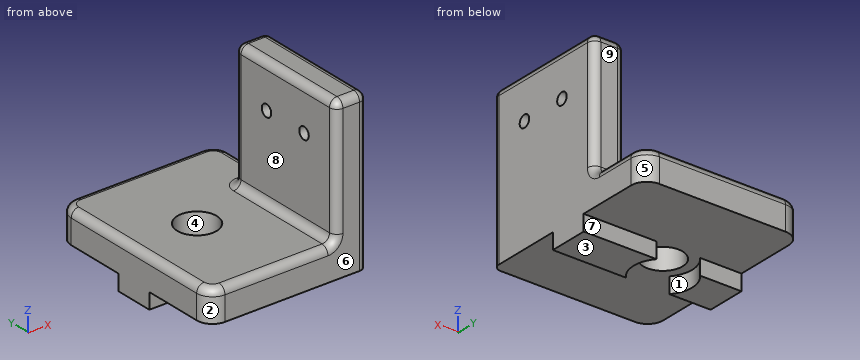
from build123d import *

# Parameters (mm, degrees)
SKETCH1_W           = 31.75
SKETCH1_H           = 38.1
BOSS_EXTRUDE1_DEPTH = 6.35
SKETCH2_W           = 6.35
SKETCH2_H           = 25.4
BOSS_EXTRUDE2_DEPTH = 25.4
SKETCH3_R           = 1.2
CUT_EXTRUDE1_DEPTH  = 7.35
SKETCH4_R           = 3.96875
CUT_EXTRUDE2_DEPTH  = 7.35
SKETCH5_W           = 3.18
SKETCH5_H           = 7.8
BOSS_EXTRUDE3_DEPTH = 31.75
FILLET1_R           = 3.175
FILLET2_R           = 1.5
CUT_EXTRUDE3_DEPTH  = 4.18
SKETCH7_R           = 5.866318131
CUT_EXTRUDE4_DEPTH  = 3.18


with BuildPart() as part:
    # Sketch1 → Boss-Extrude1 (new body)
    with BuildSketch(Plane.XY):
        with Locations((15.875, 19.05)):
            Rectangle(SKETCH1_W, SKETCH1_H)
    extrude(amount=BOSS_EXTRUDE1_DEPTH)

    # Sketch2 → Boss-Extrude2 (add)
    with BuildSketch(Plane.XY.offset(6.35)):
        with Locations((28.575, 12.7)):
            Rectangle(SKETCH2_W, SKETCH2_H)
    extrude(amount=BOSS_EXTRUDE2_DEPTH)

    # Sketch3 → Cut-Extrude1 (cut, through all)
    with BuildSketch(Plane.ZY.offset(-25.4)):
        with Locations((22.95, 17.45)):
            Circle(SKETCH3_R)
        with Locations((22.95, 7.95)):
            Circle(SKETCH3_R)
    extrude(amount=-CUT_EXTRUDE1_DEPTH, mode=Mode.SUBTRACT)

    # Sketch4 → Cut-Extrude2 (cut, through all)
    with BuildSketch(Plane.XY.offset(6.35)):
        with Locations((12.7, 19.05)):
            Circle(SKETCH4_R)
    extrude(amount=-CUT_EXTRUDE2_DEPTH, mode=Mode.SUBTRACT)

    # Sketch5 → Boss-Extrude3 (add)
    with BuildSketch(Plane.ZY):
        with Locations((-1.59, 19.05)):
            Rectangle(SKETCH5_W, SKETCH5_H)
    extrude(amount=-BOSS_EXTRUDE3_DEPTH)

    # Fillet1
    fillet1_edges = [part.edges().sort_by_distance(p)[0] for p in [
        (0, 0, 3.175),
        (0, 38.1, 3.175),
        (31.75, 38.1, 3.175),
    ]]
    fillet(fillet1_edges, radius=FILLET1_R)

    # Fillet2
    fillet2_edges = [part.edges().sort_by_distance(p)[0] for p in [
        (31.75, 30.1625, 6.35),
        (28.575, 0, 31.75),
        (25.4, 0, 19.05),
        (28.575, 25.4, 6.35),
        (31.75, 25.4, 19.05),
        (25.4, 12.7, 31.75),
        (25.4, 25.4, 19.05),
        (31.75, 12.7, 31.75),
        (28.575, 25.4, 31.75),
        (25.4, 12.7, 6.35),
        (15.875, 38.1, 6.35),
        (14.2875, 0, 6.35),
        (0, 19.05, 6.35),
        (0.92993597, 0.92993597, 6.35),
        (0.92993597, 37.17006403, 6.35),
        (30.82006403, 37.17006403, 6.35),
        (31.75, 0, 15.875),
    ]]
    fillet(fillet2_edges, radius=FILLET2_R)

    # Sketch6 → Cut-Extrude3 (cut, through all)
    with BuildSketch(Plane.XY):
        with BuildLine():
            Line((13.435511089, 22.95), (11.964488911, 22.95))
            ThreePointArc((11.964488911, 22.95), (8.73125, 19.05), (11.964488911, 15.15))
            Line((11.964488911, 15.15), (13.435511089, 15.15))
            ThreePointArc((13.435511089, 15.15), (16.66875, 19.05), (13.435511089, 22.95))
        make_face()
    extrude(amount=-CUT_EXTRUDE3_DEPTH, mode=Mode.SUBTRACT)

    # Sketch7 → Cut-Extrude4 (cut)
    with BuildSketch(Plane(origin=(0, 0, 0), x_dir=(-1, 0, 0), z_dir=(0, 0, -1))):
        with Locations((-12.7, 19.05)):
            Circle(SKETCH7_R)
    extrude(amount=CUT_EXTRUDE4_DEPTH, mode=Mode.SUBTRACT)


solid = part.part
Design review of the part built by this model. Coordinates are the model's own, in mm. Face numbers are marked on the shaded views. A direction names the side the tool comes from. Coordinates: 2 decimals unless noted, no trailing zeros. Order: outer loops, then holes, each group sorted by start corner. A loop starts at its lowest first (then second) coordinate and runs counter-clockwise, first axis right, second up. Notation, with made-up numbers: M 63,13 L 76,13 A34 ccw 76,52 Z; hole C -29,70.25 d11. An arc over 180 degrees is marked long. Use a Markdown table: item, result.
(1) Wall thickness on probe 1 along Y at (x, z) = (27.75, 22.95); probe 2 along Y at (x, z) = (13, 2); probe 3 along X at (y, z) = (19.05, 4.75): over which ranges is each line inside the solid? List them lowest first.
Worked answers:
| item | result |
|---|---|
| probe 1 | y = 0 to 6.75, 9.15 to 16.25, 18.65 to 25.4 |
| probe 2 | y = 0 to 15.09, 23.01 to 38.1 |
| probe 3 | x = 0 to 8.73, 16.67 to 31.75 |
(2) For P1, Ø7, axis at x = 12.7, y = 19.05, coming from the +Z side; P2, Ø2, axis at x = 10.5, y = 16.5, coming from the -Z side; P3, Ø6.5, axis at y = 9.5, z = 20, coming from the -X side; P4, Ø1.6, axis at x = 22, z = -1, coming from the +Y side, all flat-tipped, find the tip position at first contact; note any pin that passes through.
Worked answers:
| item | result |
|---|---|
| P1 | passes through |
| P2 | stops at z = 0 |
| P3 | stops at x = 25.4 |
| P4 | stops at y = 22.95 |
(3) Draft analysis for pull direction X (two halves, no side actions). For the marked faces 1, 2, 3 and 4, state which applies: released by +X, released by -X, zero draft, split by the parting line, or undercut.
Worked answers:
| item | result |
|---|---|
| face 1 | undercut |
| face 2 | released by -X |
| face 3 | zero draft |
| face 4 | undercut |
(4) Add section D-D (y = 17.45). Give the boundary of the cut face in (x, z).
Worked answers:
| item | result |
|---|---|
| outline | M 0,-3.18 L 7.06,-3.18 L 7.06,0 L 9.07,0 L 9.07,6.35 L 1.5,6.35 A1.5 ccw 0,4.85 Z; M 16.33,0 L 18.34,0 L 18.34,-3.18 L 31.75,-3.18 L 31.75,21.75 L 25.4,21.75 L 25.4,7.85 A1.5 cw 23.9,6.35 L 16.33,6.35 Z; M 25.4,24.15 L 31.75,24.15 L 31.75,30.25 A1.5 ccw 30.25,31.75 L 26.9,31.75 A1.5 ccw 25.4,30.25 Z |
(5) For the marked faces 5, 6, 7, 8 and 9, list the 3-axis set-ups (+Z, -Z, +X, -X, +Y, -Y) from which the entire face can be reached by the end or side of a thin tool; tool diameter is ignored.
Worked answers:
| item | result |
|---|---|
| face 5 | +Z, -Z, +X, +Y |
| face 6 | +Z, -Z, +X, -X, -Y |
| face 7 | -Z, +X, -X, +Y |
| face 8 | +Z, -X, +Y, -Y |
| face 9 | +Z, +X, -X, +Y |
(6) Add section C-C (z = 22.95). Give the boundary of the cut face in (x, y), then the cut area to 3 significant figures.
Worked answers:
| item | result |
|---|---|
| outline | M 25.4,1.5 A1.5 ccw 26.9,0 L 30.25,0 A1.5 ccw 31.75,1.5 L 31.75,6.75 L 25.4,6.75 Z; M 25.4,9.15 L 31.75,9.15 L 31.75,16.25 L 25.4,16.25 Z; M 25.4,18.65 L 31.75,18.65 L 31.75,23.9 A1.5 ccw 30.25,25.4 L 26.9,25.4 A1.5 ccw 25.4,23.9 Z |
| area | 129 mm2 |
(7) Add section B-B (y = 7.95). Give the boundary of the cut face in (x, z).
Worked answers:
| item | result |
|---|---|
| outline | M 0,0 L 31.75,0 L 31.75,21.75 L 25.4,21.75 L 25.4,7.85 A1.5 cw 23.9,6.35 L 1.5,6.35 A1.5 ccw 0,4.85 Z; M 25.4,24.15 L 31.75,24.15 L 31.75,30.25 A1.5 ccw 30.25,31.75 L 26.9,31.75 A1.5 ccw 25.4,30.25 Z |
